Autodesk Inventor part; units mm, degrees
ref_plane "bolt_to_nut_XY" through (10, 0, 0) normal (1, 0, 0) x (0, 0, -1)
ref_plane "bolt_to_nut_YZ" through (10, 0, 0) normal (0, 0, -1) x (0, 1, 0)
ref_plane "bolt_to_nut_ZX" through (10, 0, 0) normal (0, 1, 0) x (1, 0, 0)
sketch "Sketch_1" plane through (0, 0, 0) normal (0, 0, 1) x (1, 0, 0)
  line L0 (10, 0) -> (-4, 0)
  line L1 (-4, 0) -> (-4, 3.1)
  line L2 (-4, 3.1) -> (-3.6, 3.5)
  line L3 (-3.6, 3.5) -> (0, 3.5)
  line L4 (0, 3.5) -> (0, 2)
  line L5 (0, 2) -> (9.5705, 2)
  line L6 (9.5705, 2) -> (10, 1.5705)
  line L7 (10, 1.5705) -> (10, 0)
  line L8 (10, 0) -> (-4, 0)
revolve "Revolution1" add sketch "Sketch_1" angle 360 about axis through (10, 0, 0) along (1, 0, 0)
thread "Thread1"
sketch "Sketch2" plane through (-4, 0, 0) normal (-1, 0, 0) x (0, 0, 1)
  point P0 (0, 0)
hole "Hole1" at (-4, 0, 0) direction (1, 0, 0) diameter 3 depth 2 tip angle 150
sketch "Sketch_3" plane through (-4, 0, 0) normal (1, 0, 0) x (0, 0, -1)
  line L0 (-1.5, -0.866) -> (0, -1.7321)
  line L1 (0, -1.7321) -> (1.5, -0.866)
  line L2 (1.5, -0.866) -> (1.5, 0.866)
  line L3 (1.5, 0.866) -> (0, 1.7321)
  line L4 (0, 1.7321) -> (-1.5, 0.866)
  line L5 (-1.5, 0.866) -> (-1.5, -0.866)
extrude "Extrusion1" cut sketch "Sketch_3" along normal blind 2
ref_plane "bolt_to_nut_XY" through (10, 0, 0) normal (1, 0, 0) x (0, 0, -1)
ref_plane "bolt_to_nut_YZ" through (10, 0, 0) normal (0, 0, -1) x (0, 1, 0)
ref_plane "bolt_to_nut_ZX" through (10, 0, 0) normal (0, 1, 0) x (1, 0, 0)
ref_plane "screw1_XY" through (0, 0, 0) normal (1, 0, 0) x (0, 0, -1)
ref_plane "screw1_YZ" through (0, 0, 0) normal (0, 0, -1) x (0, 1, 0)
ref_plane "screw1_ZX" through (0, 0, 0) normal (0, 1, 0) x (1, 0, 0)
properties part number "CB4-10" material "鋼、炭素鋼"
The listing builds one solid part. Answer for the finished solid, in the listing's coordinates (mm). A direction names the side the tool comes from. Give positions to 0.01 mm unless a question says otherwise; leave off trailing zeros. Order: outer loops, then holes, each group sorted by start corner. A loop starts at its lowest first (then second) coordinate and runs counter-clockwise, first axis right, second up. Notation, with made-up numbers: (-39, -22) - (-8, -22) arc R14 ccw to (-8, -4) - close; hole circle Ø2 at (46.5, 34). An arc over 180 degrees is marked (long way). One line per item, written item: value. Start each with the question number.
1) A cutting plane is placed at B-B on x = 8. Give the vertices of the cut face in (y, z).
2) The mould has two halves that part along Y. Classify faces 1 (the face through (-4, 1.3, -1.3)), 2 (the face through (-3.014, -1.293, 0.76)), 3 (the face through (-1.775, 3.233, -1.341)): released by +Y, released by -Y, zero draft, split by the parting line, or undercut.
3) A tool of negligible diameter and unlimited length cuts with its end or side. For faces 4 (the face through (10, 0, 0)), 5 (the face through (5, 0, -2)), 6 (the face through (-3.014, 1.293, -0.76)), from which of +Z, -Z, +X, -X, +Y, -Y can it reach the whole face along a straight path? Write none if from no direction.
4) A cutting plane is placed at A-A on x = -2.5. Give the vertices of the cut face in (y, z).
5) Given pin 1 Ø1 at (x, y) = (-1, -1) entering from +Z; pin 2 Ø3 at (x, y) = (2.5, -2) entering from +Z; pin 3 Ø2 at (x, z) = (3, 2.5) entering from -Y, each flat-ended and moving along its own axis, determine where each tip first touches the part or whether it passes through.
6) Find the intervals of material crossed by L1, parallel to X at y = -0.5, z = 3; L2, parallel to Y at x = -0.5, z = 0.5; L3, parallel to Z at x = 3.5, y = -0.25, in increasing order.
Answer sheet:
1. outline: circle Ø4 at (0, 0)
2. face 1: zero draft
2. face 2: undercut
2. face 3: split by the parting line
3. face 4: +Z, -Z, +X, +Y, -Y
3. face 5: +X
3. face 6: -X
4. outline: circle Ø7 at (0, 0); hole (-1.73, 0) - (-0.87, -1.5) - (0.87, -1.5) - (1.73, 0) - (0.87, 1.5) - (-0.87, 1.5) - close
5. pin 1: stops at z = 3.46
5. pin 2: stops at z = 1.94
5. pin 3: stops at y = -1.32
6. L1: x = -4 to 0
6. L2: y = -3.46 to 3.46
6. L3: z = -1.98 to 1.98
